```python
from build123d import *

# Parameters (mm, degrees)
F2_W     = 38.898766
F2_H     = 7.372967
F3_DEPTH = 3.81
F4_R     = 1.58321
F5_DEPTH = 22.86


with BuildPart() as f1:
    # F0 (on Front) → F1 (revolve)
    with BuildSketch(Plane.XZ):
        with BuildLine():
            Line((0, 47.11812), (0, 0))
            ThreePointArc((0, 0), (23.55906, 23.55906), (0, 47.11812))
        make_face()
    revolve(axis=Axis((0, 0, 23.55906), (0, 0, 1)))

    # F2 (on Front) → F3 (join, symmetric)
    with BuildSketch(Plane.XZ):
        with Locations((-1.117459, 44.860396)):
            Rectangle(F2_W, F2_H)
    extrude(amount=F3_DEPTH, both=True)

    # F4 (on Right) → F5 (cut, symmetric)
    with BuildSketch(Plane.YZ):
        with Locations((0, 44.889353)):
            Circle(F4_R)
    extrude(amount=F5_DEPTH, both=True, mode=Mode.SUBTRACT)


solid = f1.part
```
Input: part model. Units: mm. Frame: model coordinates. A direction names the side the tool comes from. Round coordinates to 2 decimals unless told otherwise and drop trailing zeros. Loops run counter-clockwise (first coordinate to the right, second up) from the corner with the lowest first, then second, coordinate; pieces in that order, holes last. Notation, with made-up numbers: M 86,89.25 L 140,89.25 A37 cw 140,128.25 Z; hole C 21.5,54 d5. An arc over 180 degrees is marked long. Answer in a Markdown table with one row per item. Add a question column.
1. Section B-B (x = -16). Output: boundary loops of the cut face in (y, z).
2. Section D-D (z = 29.5). Output: boundary loops of the cut face in (x, y), and give its area (3 significant figures).
3. Section A-A (y = 0). Output: boundary loops of the cut face in (x, z).
4. Mould query, pull axis Z, two halves, no side actions, for faces 5 (the face through (17, 0, 41.174)), 6 (the face through (-1, 0, 48.547)), 7 (the face through (18.332, 0, 43)). Classes: released by +Z, released by -Z, zero draft, split by the parting line, or undercut.
5. Section C-C (x = -2.5). Output: boundary loops of the cut face in (y, z).
6. Contact query for flat-ended pins moving along their axis: pin 1 (8 mm diameter, centred on x = -7.5, z = 28.5, fed in from -Y); pin 2 (2 mm diameter, centred on y = -1, z = 44, fed in from -X); pin 3 (6 mm diameter, centred on y = -11, z = 12, fed in from +X). Output: stop coordinate, or through.
7. Set-up query: faces 1 (the face through (-0.845, -0.343, 43.344)), 2 (the face through (-1, -3.81, 47)), 3 (the face through (-20.567, 0, 43)), 4 (the face through (-1, 3.81, 47)). Return all of +Z, -Z, +X, -X, +Y, -Y with unobstructed straight access to the full face (end or side cutting, diameter ignored); none if empty.
8. Ray query, probe 1 along Z at (x, y) = (10, 0); probe 2 along X at (y, z) = (-3.5, 43); probe 3 along X at (y, z) = (-16.5, 27.5). Return the intervals inside material, ascending.
Values follow:
| question | item | result |
|---|---|---|
| 1 | outline | C 0,23.56 d34.58; M -3.81,41.17 L 3.81,41.17 L 3.81,48.55 L -3.81,48.55 Z; hole C 0,44.89 d3.17 |
| 2 | outline | C 0,0 d45.6 |
| 2 | area | 1,630 mm^2 |
| 3 | outline | M -20.57,41.17 L -15.64,41.17 A23.56 ccw long 15.64,41.17 L 18.33,41.17 L 18.33,43.31 L -20.57,43.31 Z; M -20.57,46.47 L 18.33,46.47 L 18.33,48.55 L -20.57,48.55 Z |
| 4 | face 5 | undercut |
| 4 | face 6 | released by +Z |
| 4 | face 7 | zero draft |
| 5 | outline | M -3.81,46.67 A23.43 ccw long 3.81,46.67 L 3.81,48.55 L -3.81,48.55 Z; hole C 0,44.89 d3.17 |
| 6 | pin 1 | y = -23.03 |
| 6 | pin 2 | x = -20.57 |
| 6 | pin 3 | x = 19.68 |
| 7 | face 1 | +X, -X |
| 7 | face 2 | +Z, -Y |
| 7 | face 3 | +Z, -X, +Y, -Y |
| 7 | face 4 | +Z, +Y |
| 8 | probe 1 | 2.23 to 43.31, 46.47 to 48.55 |
| 8 | probe 2 | -20.57 to 18.33 |
| 8 | probe 3 | -16.35 to 16.35 |
